Autodesk Inventor part; units mm, degrees
ref_plane "Start Plane" through (0, 0, 8.6865) normal (0, 0, 1) x (1, 0, 0)
ref_plane "End Plane" through (0, 0, 71.9966) normal (0, 0, 1) x (1, 0, 0)
ref_plane "Work Plane5" through (1.8939, -115, 12.0587) normal (0.4394, 0, -0.8983) x (-0.8983, 0, -0.4394)
ref_plane "Start Plane" through (0, 0, 8.6865) normal (0, 0, 1) x (1, 0, 0)
ref_plane "End Plane" through (0, 0, 71.9966) normal (0, 0, 1) x (1, 0, 0)
sketch "Sketch" plane through (0, 0, 0) normal (0, 0, 1) x (1, 0, 0)
  line L0 (5, -5) -> (-5, -5)
  line L1 (-5, -5) -> (-5, 5)
  line L2 (-5, 5) -> (5, 5)
  line L3 (5, 5) -> (5, -5)
  line L4 (-6, 0) -> (8, 0) construction
  line L5 (0, -30) -> (0, 40) construction
  line L6 (0, 54) -> (0, -44) construction
  line L7 (-9.2, 0) -> (13.2, 0) construction
  dimension "d0" = 10
  dimension "d1" = 10
  dimension "d4" = 5
  dimension "d5" = 5
extrude "Body" add sketch "Sketch" along normal up to surface (63.3101 mm away) from surface at 8.6865
sketch "Sketch3" plane through (0, 0, 0) normal (0, 0, 1) x (1, 0, 0)
  line L0 (0, 0) -> (10, 0)
ref_plane "Work Plane3" through (0, 0, 0) normal (0, -1, 0) x (1, 0, 0)
sketch "Sketch4" plane through (0, 0, 0) normal (0, -1, 0) x (1, 0, 0)
  line L0 (-2, 8.6865) -> (12, 8.6865)
  line L1 (-2, 71.9966) -> (12, 71.9966)
  dimension "d9" = 63.3101
ref_plane "Work Plane5" through (1.8939, -115, 12.0587) normal (0.4394, 0, -0.8983) x (-0.8983, 0, -0.4394)
split "Split2" plane through (1.8939, -115, 12.0587) removes the side toward (0.4394, 0, -0.8983)
ref_plane "Work Plane6" through (-0.1986, 5, 71.79) normal (-0.0397, 0, 0.9992) x (0.9992, 0, 0.0397)
split "Split3" plane through (-0.1986, 5, 71.79) removes the side toward (-0.0397, 0, 0.9992)
equation "\"d0\" = G_W"
equation "\"d1\" = G_H"
equation "\"d4\" = 0.5 * d1"
equation "\"d5\" = 0.5 * d0"
equation "\"d2\" = G_L"
equation "\"G_W\" = 10"
equation "\"G_H\" = 10"
equation "\"G_L\" = d9"
equation "\"G_OFFSET_START\" = -8.68648"
equation "\"G_OFFSET_END\" = 5.20268"
equation "\"d6\" = -G_OFFSET_START"
equation "\"d7\" = G_OFFSET_END + B_L"
equation "\"B_L\" = 66.7939"
properties part number "ISO 1035/2 - 10 x 10 - 63.31" material "Steel, Mild"
Check sheet for the modelled part. Datum: model origin and axes. Units: mm. Round coordinates to 2 decimals unless told otherwise and drop trailing zeros. Order: outer loops, then holes, each group sorted by start corner. A loop starts at its lowest first (then second) coordinate and runs counter-clockwise, first axis right, second up. Notation, with made-up numbers: M -23,56 L -11,56 A26 ccw -11,84 Z; hole C 52,-3 d2. An arc over 180 degrees is marked long. One line per item, written item: value. Start each with the question number.
1. Gauge pin test, flat ends, axial feed: P1, Ø4, axis at x = -3.5, y = -1.5, coming from the -Z side; P2, Ø1, axis at x = 1.5, y = 4, coming from the +Z side. Record the tip position at first contact, or that the pin passes through.
2. Section check B-B on x = 2.75. Enter the section's corners in (y, z), and give its area (3 significant figures).
3. Section check A-A on y = -0.25. Enter the section's corners in (x, z).
4. Scan lines: line 1 along Z through (x, y) = (3.25, -4); line 2 along Z through (x, y) = (1, -0.5); line 3 along X through (y, z) = (-2.75, 12.5). Record each from-to range of solid material in increasing order.
Results found:
1. P1: z = 8.69
1. P2: z = 71.88
2. outline: M -5,12.48 L 5,12.48 L 5,71.91 L -5,71.91 Z
2. area: 594 mm^2
3. outline: M -5,8.69 L 5,13.58 L 5,72 L -5,71.6 Z
4. line 1: 12.72 to 71.93
4. line 2: 11.62 to 71.84
4. line 3: -5 to 2.8
